For this review, take the finished solid that the model builds, in its own axes (mm). Round coordinates to 2 decimals unless told otherwise and drop trailing zeros. Write each loop counter-clockwise with the first axis right and the second up, starting at its lowest first coordinate (ties: lowest second). Pieces come first, ordered by that corner, then holes. Notation, with made-up numbers: (-19.5, 31.5) -> (11.5, 31.5) arc R18 cw to (11.5, 65.5) -> close; hole circle Ø10 at (4.25, -39). An arc over 180 degrees is marked (long way). Answer in a Markdown table with one row per item.
from build123d import *

# Parameters (mm, degrees)
F1_DEPTH = 1.524
F2_W     = 6.858
F2_H     = 4.572
F3_DEPTH = 0.254
F4_W     = 6.858
F4_H     = 4.572
F5_DEPTH = 0.254


with BuildPart() as f1:
    # F0 (on Top) → F1 (new body)
    with BuildSketch(Plane.XY):
        with BuildLine():
            Line((-53.369354, -22.832613), (-53.369354, 5.281494))
            Line((-53.369354, 5.281494), (-62.412295, 5.281494))
            ThreePointArc((-62.412295, 5.281494), (-61.67148, -8.969847), (-65.058701, -22.832613))
            Line((-65.058701, -22.832613), (-53.369354, -22.832613))
        make_face()
    extrude(amount=F1_DEPTH)

    # F2 (on face) → F3 (join)
    with BuildSketch(Plane.XY.offset(1.524)):
        with Locations((-56.798354, 2.995494)):
            Rectangle(F2_W, F2_H)
        with Locations((-56.798354, -20.546613)):
            Rectangle(F2_W, F2_H)
    extrude(amount=F3_DEPTH)

    # F4 (on face) → F5 (join)
    with BuildSketch(Plane(origin=(0, 0, 0), x_dir=(1, 0, 0), z_dir=(0, 0, -1))):
        with Locations((-56.798354, -2.995494)):
            Rectangle(F4_W, F4_H)
        with Locations((-56.798354, 20.546613)):
            Rectangle(F4_W, F4_H)
    extrude(amount=F5_DEPTH)


solid = f1.part
1) Clearance check with a flat-ended pin moving along its axis: pin 1 Ø6 at (x, y) = (-57, -14.5) entering from +Z. State where the tip first meets the part, or that it passes through.
Solved:
| item | result |
|---|---|
| pin 1 | z = 1.52 |
2) For line 1 (Z direction, x = -55.25, y = -11.5); line 2 (X direction, y = -2.75, z = 0.4); line 3 (X direction, y = -7.75, z = 1.2), list the stretches that pass through material, from the lowest coordinate up. Write a range as [from, to].
Solved:
| item | result |
|---|---|
| line 1 | [0, 1.52] |
| line 2 | [-61.48, -53.37] |
| line 3 | [-61.57, -53.37] |
3) Consider section D-D on z = 1. State the section outline as (x, y) points, then the cut area to 3 significant figures.
Solved:
| item | result |
|---|---|
| outline | (-65.06, -22.83) -> (-53.37, -22.83) -> (-53.37, 5.28) -> (-62.41, 5.28) arc R49.12 cw to start |
| area | 252 mm² |
4) Consider section B-B on x = -55.5. State the section outline as (y, z) points.
Solved:
| item | result |
|---|---|
| outline | (-22.83, -0.25) -> (-18.26, -0.25) -> (-18.26, 0) -> (0.71, 0) -> (0.71, -0.25) -> (5.28, -0.25) -> (5.28, 1.78) -> (0.71, 1.78) -> (0.71, 1.52) -> (-18.26, 1.52) -> (-18.26, 1.78) -> (-22.83, 1.78) -> close |
5) Mouldability with a two-part tool opening along Y and no side actions: class faces 1 (the flat face through (-58, 5.281, 1)), 2 (the flat face through (-58, -12, 0)), 3 (the cylindrical face through (-61.653, -8.77, 0.751)), 4 (the flat face through (-57, -21, -0.254)) as pulls with the +Y half, pulls with the -Y half, needs draft (parallel to the pull), parting line crosses it, or undercut.
Solved:
| item | result |
|---|---|
| face 1 | pulls with the +Y half |
| face 2 | undercut |
| face 3 | undercut |
| face 4 | needs draft |
6) Consider section C-C on y = 3.5. State the section outline as (x, z) points.
Solved:
| item | result |
|---|---|
| outline | (-62.09, 0) -> (-60.23, 0) -> (-60.23, -0.25) -> (-53.37, -0.25) -> (-53.37, 1.78) -> (-60.23, 1.78) -> (-60.23, 1.52) -> (-62.09, 1.52) -> close |
7) Consider section A-A on x = -61.75. State the section outline as (y, z) points.
Solved:
| item | result |
|---|---|
| outline | (-22.83, 0) -> (-9.74, 0) -> (-9.74, 1.52) -> (-22.83, 1.52) -> close; (1.01, 0) -> (5.28, 0) -> (5.28, 1.52) -> (1.01, 1.52) -> close |
